Source: CAD feature listing. Evaluate the final solid. Frame: model axes, mm. A direction names the side the tool comes from. Round coordinates to 2 decimals unless told otherwise and drop trailing zeros. Loops run counter-clockwise (first coordinate to the right, second up) from the corner with the lowest first, then second, coordinate; pieces in that order, holes last. Notation, with made-up numbers: (24.5, 80) - (68.5, 80) arc R33 cw to (68.5, 115) - close; hole circle Ø3 at (21, 19.5). An arc over 180 degrees is marked (long way). One line per question, with ' | ' between items.
from build123d import *

# Parameters (mm, degrees)
SKETCH_W        = 150
SKETCH_H        = 56
SKETCH_R        = 8
SKETCH_W_2      = 72
SKETCH_H_2      = 25
PAD_DEPTH       = 3
PAD001_DEPTH    = 4
SKETCH002_R     = 1.5
POCKET_DEPTH    = 5
SKETCH003_R     = 1
POCKET001_DEPTH = 5
FILLET_R        = 2


with BuildPart() as part:
    # Sketch → Pad (new body)
    with BuildSketch(Plane.XY):
        with Locations((75, 28)):
            Rectangle(SKETCH_W, SKETCH_H)
        with Locations((18, 16.5)):
            Circle(SKETCH_R, mode=Mode.SUBTRACT)
        with Locations((18, 39.5)):
            Circle(SKETCH_R, mode=Mode.SUBTRACT)
        with Locations((132, 16.5)):
            Circle(SKETCH_R, mode=Mode.SUBTRACT)
        with Locations((132, 39.5)):
            Circle(SKETCH_R, mode=Mode.SUBTRACT)
        with Locations((75, 28)):
            Rectangle(SKETCH_W_2, SKETCH_H_2, mode=Mode.SUBTRACT)
    extrude(amount=PAD_DEPTH)

    # Sketch001 (on Face14 of Pad) → Pad001 (join)
    with BuildSketch(Plane.XY.offset(3)):
        Polygon((39, 15.5), (111, 15.5), (116, 15.5), (116, 8.5), (109, 8.5), (109, 14.5), (34, 14.5), (34, 45.5), (111, 45.5), (116, 45.5), (116, 40.5), (111, 40.5), (39, 40.5), align=None)
    extrude(amount=PAD001_DEPTH)

    # Sketch002 (on Face5 of Pad001) → Pocket (cut)
    with BuildSketch(Plane.XY.offset(3)):
        with Locations((3, 53)):
            Circle(SKETCH002_R)
        with Locations((147, 53)):
            Circle(SKETCH002_R)
        with Locations((3, 3)):
            Circle(SKETCH002_R)
        with Locations((147, 3)):
            Circle(SKETCH002_R)
    extrude(amount=-POCKET_DEPTH, mode=Mode.SUBTRACT)

    # Sketch003 (on Face32 of Pocket) → Pocket001 (cut)
    with BuildSketch(Plane.XY.offset(7)):
        with Locations((37, 43)):
            Circle(SKETCH003_R)
        with Locations((113, 43)):
            Circle(SKETCH003_R)
        with Locations((113, 12)):
            Circle(SKETCH003_R)
    extrude(amount=-POCKET001_DEPTH, mode=Mode.SUBTRACT)

    # Fillet
    fillet_edges = [part.edges().sort_by_distance(p)[0] for p in [
        (0, 0, 1.5),
        (0, 56, 1.5),
        (150, 0, 1.5),
        (150, 56, 1.5),
    ]]
    fillet(fillet_edges, radius=FILLET_R)


solid = part.part
1. Section query B-B, the plane x = 95. Return loops of the section in (y, z).
Worked out:
outline: (0, 0) - (15.5, 0) - (15.5, 7) - (14.5, 7) - (14.5, 3) - (0, 3) - close; (40.5, 0) - (56, 0) - (56, 3) - (45.5, 3) - (45.5, 7) - (40.5, 7) - close
2. Section query D-D, the plane x = 11.5. Return loops of the section in (y, z).
Worked out:
outline: (0, 0) - (11.84, 0) - (11.84, 3) - (0, 3) - close; (21.16, 0) - (34.84, 0) - (34.84, 3) - (21.16, 3) - close; (44.16, 0) - (56, 0) - (56, 3) - (44.16, 3) - close
3. Material intervals for probe 1 along Y at (x, z) = (147, 1.2); probe 2 along Y at (x, z) = (18, 2.3); probe 3 along Y at (x, z) = (67.5, 3.75), sorted ascending.
Worked out:
probe 1: y = 0 to 1.5, 4.5 to 51.5, 54.5 to 56 | probe 2: y = 0 to 8.5, 24.5 to 31.5, 47.5 to 56 | probe 3: y = 14.5 to 15.5, 40.5 to 45.5
4. Section query C-C, the plane y = 38. Return loops of the section in (x, z).
Worked out:
outline: (0, 0) - (10.14, 0) - (10.14, 3) - (0, 3) - close; (25.86, 0) - (39, 0) - (39, 7) - (34, 7) - (34, 3) - (25.86, 3) - close; (111, 0) - (124.14, 0) - (124.14, 3) - (111, 3) - close; (139.86, 0) - (150, 0) - (150, 3) - (139.86, 3) - close
5. Access query for faces 1 (the flat face through (39, 28, 3)), 2 (the flat face through (74, 0, 1)), 3 (the flat face through (76, 45.5, 5)), 4 (the flat face through (34, 30, 5)). Directions: +Z, -Z, +X, -X, +Y, -Y. A direction counts if a zero-diameter tool reaches every point of the face in a straight line with its end or side. Return the directions, or none.
Worked out:
face 1: +Z, -Z | face 2: +Z, -Z, +X, -X, -Y | face 3: +Z, +X, -X, +Y | face 4: +Z, -X, +Y, -Y
6. Mould query, pull axis X, two halves, no side actions, for faces 5 (the flat face through (116, 12, 5)), 6 (the flat face through (77, 40.5, 3)), 7 (the flat face through (109, 11, 5)). Classes: released by +X, released by -X, zero draft, split by the parting line, or undercut.
Worked out:
face 5: released by +X | face 6: undercut | face 7: released by -X
7. Contact query for flat-ended pins moving along their axis: P1, Ø2, axis at y = 12, z = 6, coming from the +X side; P2, Ø1, axis at x = 72.5, z = 5.5, coming from the +Y side; P3, Ø1.6, axis at x = 37, y = 43, coming from the +Z side. Output: stop coordinate, or through.
Worked out:
P1: stops at x = 116 | P2: stops at y = 45.5 | P3: stops at z = 2
8. Section query A-A, the plane x = 132. Return loops of the section in (y, z), plus the area to 3 significant figures.
Worked out:
outline: (0, 0) - (8.5, 0) - (8.5, 3) - (0, 3) - close; (24.5, 0) - (31.5, 0) - (31.5, 3) - (24.5, 3) - close; (47.5, 0) - (56, 0) - (56, 3) - (47.5, 3) - close | area: 72.0 mm2
